The figure shows three views and two pictorial views of one solid part (mm, origin at its lowest corner). Answer the questions. Coordinates: 2 decimals unless noted, no trailing zeros. Order: outer loops, then holes, each group sorted by start corner. A loop starts at its lowest first (then second) coordinate and runs counter-clockwise, first axis right, second up. Notation, with made-up numbers: (19.5, 58.25) -> (38.5, 58.25) arc R22 cw to (38.5, 68.25) -> close; hole circle Ø3 at (24.25, 56). An arc over 180 degrees is marked (long way). Write item = value, one per line. Start each with the question number.
Q1. Straight lines are drawn through the part: L1, parallel to X at y = 13.5, z = 1.45 (1 decimal); L2, parallel to X at y = 14.75, z = 1.7 (1 decimal); L3, parallel to Y at x = 12.5, z = 0.75. For each, find the intervals that lie inside material, in ascending order. Write a range as from..to.
Q2. The part is cut by section A-A, the plane y = 10. Determine the outline of the cut face in (x, z).
Q3. Flat-ended cylindrical pins translate along their axes: pin 1 (1 mm diameter, centred on x = 1, z = 1, fed in from +Y); pin 2 (1 mm diameter, centred on x = 11.5, z = 1.5, fed in from -Y); pin 3 (1 mm diameter, centred on x = 42.5, z = 1, fed in from -Y). Find the tip coordinate at first contact, or state that the pin passes through.
Q4. The part is cut by section B-B, the plane x = 21.75. Determine the outline of the cut face in (y, z).
Q5. The part is cut by section C-C, the plane y = 3.5. Determine the outline of the cut face in (x, z).
Q6. The part is cut by section D-D, the plane x = 31. Determine the outline of the cut face in (y, z).
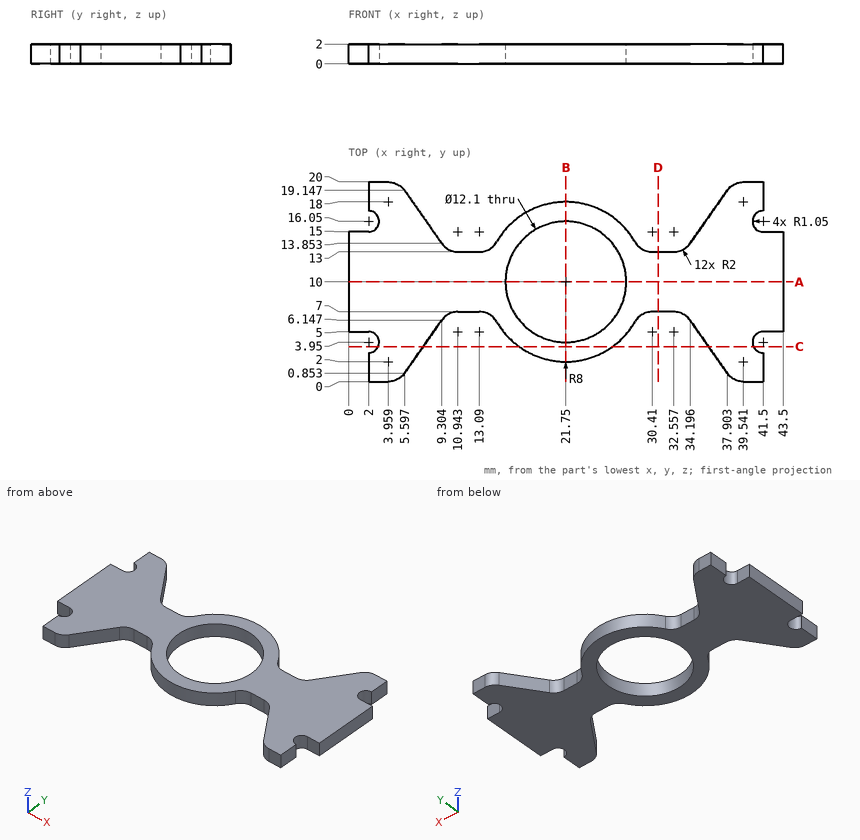
Model answer:
q1.L1 = 0..9.6, 14.4..16.8, 26.7..29.1, 33.9..43.5
q1.L2 = 0..8.7, 15.3..18, 25.5..28.2, 34.8..43.5
q1.L3 = 7..13
q2.outline = (0, 0) -> (15.7, 0) -> (15.7, 2) -> (0, 2) -> close; (27.8, 0) -> (43.5, 0) -> (43.5, 2) -> (27.8, 2) -> close
q3.pin_1 = 15
q3.pin_2 = 7
q3.pin_3 = 5
q4.outline = (2, 0) -> (3.95, 0) -> (3.95, 2) -> (2, 2) -> close; (16.05, 0) -> (18, 0) -> (18, 2) -> (16.05, 2) -> close
q5.outline = (2.95, 0) -> (7.45, 0) -> (7.45, 2) -> (2.95, 2) -> close; (17.09, 0) -> (26.41, 0) -> (26.41, 2) -> (17.09, 2) -> close; (36.05, 0) -> (40.55, 0) -> (40.55, 2) -> (36.05, 2) -> close
q6.outline = (7, 0) -> (13, 0) -> (13, 2) -> (7, 2) -> close
